Part print with two shaded views. Sizes in mm from the minimum x, y, z corner. A direction names the side the tool comes from. Coordinates: 2 decimals unless noted, no trailing zeros. Write each loop counter-clockwise with the first axis right and the second up, starting at its lowest first coordinate (ties: lowest second). Pieces come first, ordered by that corner, then holes. Notation, with made-up numbers: (37, 27.25) - (49, 27.25) arc R27 ccw to (49, 66.25) - close; hole circle Ø4 at (-16, 17). An arc over 180 degrees is marked (long way). Answer in a Markdown table with one row per item. Add a question column.
Q1. Band-saw the part on C-C (y = 5.5). List the corners of the cut face in (x, z), and give its area (3 significant figures).
Q2. Band-saw the part on D-D (x = 45.65). List the corners of the cut face in (y, z), and give its area (3 significant figures).
Q3. Band-saw the part on B-B (z = 1). List the corners of the cut face in (x, y).
Q4. 3-axis set-ups, long thin cutter, end or side, ignore diameter. For the marked faces 1, 2 and 3: which of +Z, -Z, +X, -X, +Y, -Y reach the whole face in a straight line?
Q5. Drill centre lines: line 1 along X through (y, z) = (8.25, 1.5); line 2 along Y through (x, z) = (12.35, 3.3); line 3 along Y through (x, z) = (4, 3.25). Where is each one in solid material? Low to high. Write a range as from..to.
Q6. Band-saw the part on A-A (x = 54). List the corners of the cut face in (y, z).
Q7. Pin check, flat tips, straight feed: pin 1 (5 mm diameter, centred on x = 13, y = 16, fed in from +Z); pin 2 (1.5 mm diameter, centred on x = 34.5, z = 5, fed in from -Y); pin 3 (5 mm diameter, centred on x = 45.65, y = 9.25, fed in from -Z); pin 4 (4.5 mm diameter, centred on y = 11, z = 8, fed in from -X). Stop position of each tip, or through.
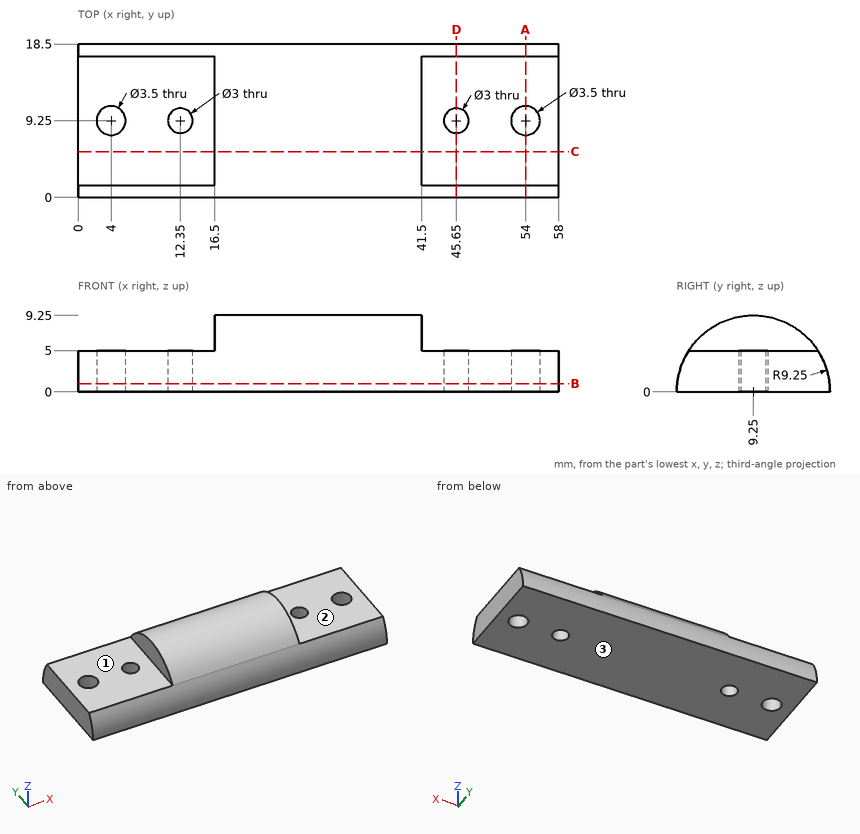
Checked values:
| question | item | result |
|---|---|---|
| 1 | outline | (0, 0) - (58, 0) - (58, 5) - (41.5, 5) - (41.5, 8.46) - (16.5, 8.46) - (16.5, 5) - (0, 5) - close |
| 1 | area | 376 mm² |
| 2 | outline | (0, 0) - (7.75, 0) - (7.75, 5) - (1.47, 5) arc R9.25 ccw to start; (10.75, 0) - (18.5, 0) arc R9.25 ccw to (17.03, 5) - (10.75, 5) - close |
| 2 | area | 72.8 mm² |
| 3 | outline | (0, 0.05) - (58, 0.05) - (58, 18.45) - (0, 18.45) - close; hole circle Ø3.5 at (4, 9.25); hole circle Ø3 at (12.35, 9.25); hole circle Ø3 at (45.65, 9.25); hole circle Ø3.5 at (54, 9.25) |
| 4 | face 1 | +Z, -X, +Y, -Y |
| 4 | face 2 | +Z, +X, +Y, -Y |
| 4 | face 3 | -Z, +X, -X, +Y, -Y |
| 5 | line 1 | x = 0..2.56, 5.44..11.23, 13.47..44.53, 46.77..52.56, 55.44..58 |
| 5 | line 2 | y = 0.61..7.75, 10.75..17.89 |
| 5 | line 3 | y = 0.59..7.5, 11..17.91 |
| 6 | outline | (0, 0) - (7.5, 0) - (7.5, 5) - (1.47, 5) arc R9.25 ccw to start; (11, 0) - (18.5, 0) arc R9.25 ccw to (17.03, 5) - (11, 5) - close |
| 7 | pin 1 | stops at z = 5 |
| 7 | pin 2 | stops at y = 1.03 |
| 7 | pin 3 | stops at z = 0 |
| 7 | pin 4 | stops at x = 16.5 |
